Source: three-view drawing plus pictorial views. Frame: mm from the lowest corner of the part. Give positions to 0.01 mm unless a question says otherwise; leave off trailing zeros. Write each loop counter-clockwise with the first axis right and the second up, starting at its lowest first coordinate (ties: lowest second). Pieces come first, ordered by that corner, then holes. Notation, with made-up numbers: (-7.5, 59.5) - (10.5, 59.5) arc R25 ccw to (10.5, 97.5) - close; hole circle Ø6 at (2, 77). An arc over 180 degrees is marked (long way). One line per question, with ' | ' between items. Start each with the question number.
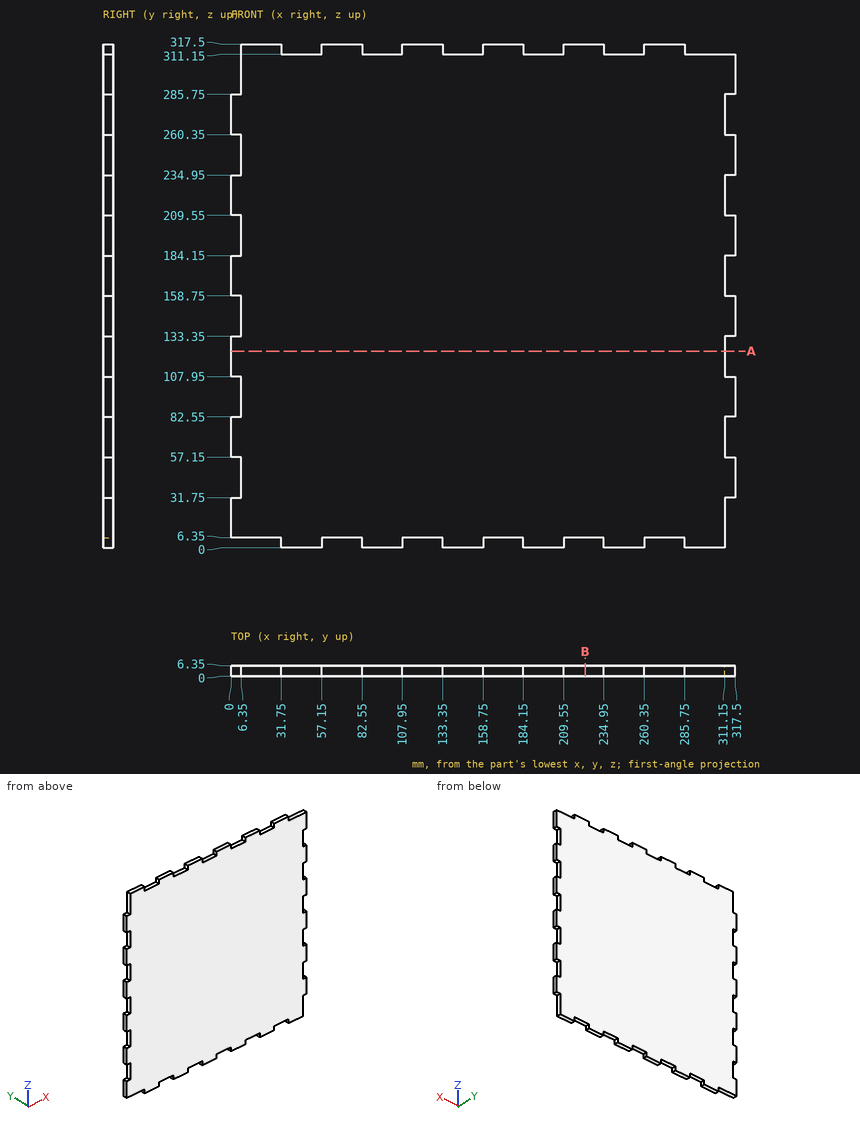
1) Section A-A, the plane z = 124. Output: boundary loops of the cut face in (x, y).
2) First-contact query: pin 1 Ø3 at (y, z) = (3.5, 145) entering from -X; pin 2 Ø3 at (x, y) = (3.5, 1.5) entering from -Z; pin 3 Ø3 at (y, z) = (1.5, 4) entering from -X; pin 4 Ø5 at (x, z) = (99.5, 153) entering from -Y. Flat tips, straight axial feed; report the tip coordinate or a pass-through.
3) Section B-B, the plane x = 223. Output: boundary loops of the cut face in (y, z), plus the area to 3 significant figures.
4) Line query: L1, parallel to Z at x = 43.5, y = 5; L2, parallel to Z at x = 122.5, y = 5.25. Output: solid intervals per line, ascending.
Answer key:
1) outline: (0, 0) - (311.15, 0) - (311.15, 6.35) - (0, 6.35) - close
2) pin 1: x = 6.35 | pin 2: z = 6.35 | pin 3: x = 31.75 | pin 4: y = 0
3) outline: (0, 6.35) - (6.35, 6.35) - (6.35, 317.5) - (0, 317.5) - close | area: 1,980 mm^2
4) L1: 0 to 311.15 | L2: 6.35 to 317.5
